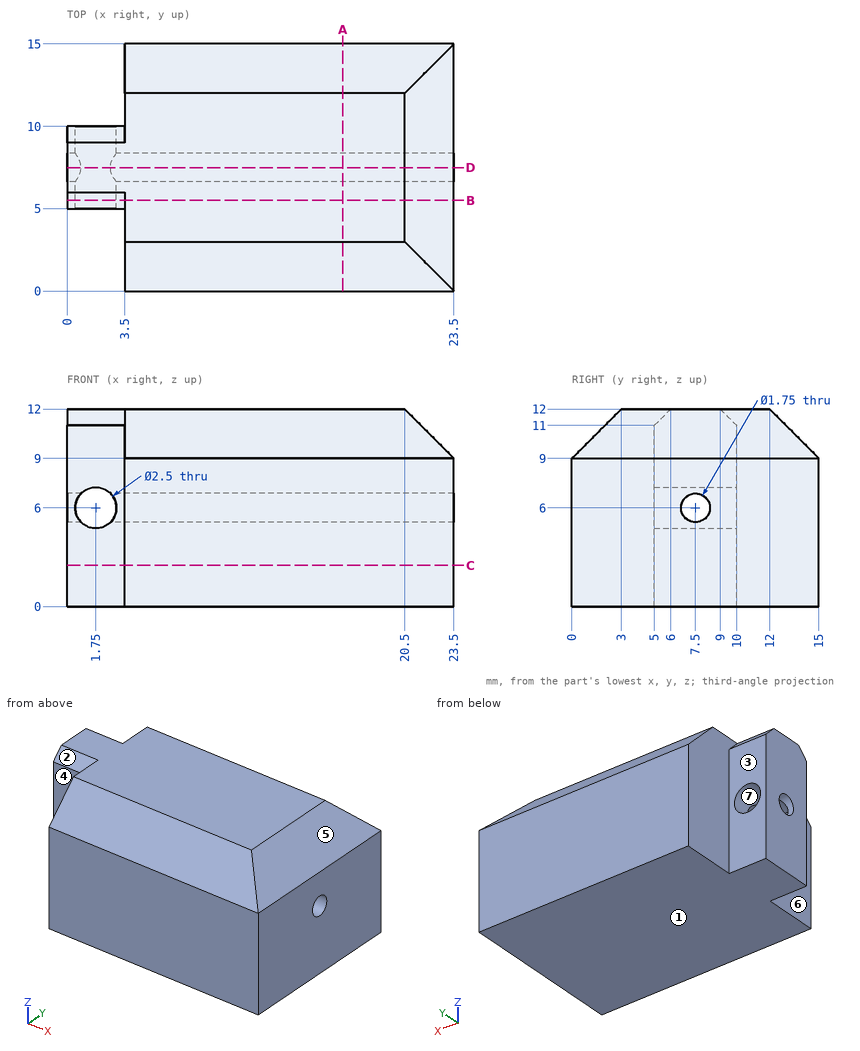
For this review, use the dimensioned drawing (mm, ordinates from the lowest corner) and the shaded views. A direction names the side the tool comes from. Coordinates: 2 decimals unless noted, no trailing zeros. Order: outer loops, then holes, each group sorted by start corner. A loop starts at its lowest first (then second) coordinate and runs counter-clockwise, first axis right, second up. Notation, with made-up numbers: (-0.75, 15) - (28.25, 15) arc R12 ccw to (28.25, 23) - close; hole circle Ø4 at (8.25, 65.5). An arc over 180 degrees is marked (long way). Answer as a JSON object with one key per item and string values. Group by question number.
1. For the marked faces 1, 2 and 3, list the 3-axis set-ups (+Z, -Z, +X, -X, +Y, -Y) from which the entire face can be reached by the end or side of a thin tool; tool diameter is ignored.
2. For probe 1 along Y at (x, z) = (15, 6) (3 decimals); probe 2 along Z at (x, y) = (0.2, 7.5) (3 decimals); probe 3 along X at (y, z) = (8.65, 6), list the stretches that pass through material, from the lowest coordinate up.
3. We need section A-A on x = 16.75. State the section outline as (y, z) points (3 decimals), then the cut area to 3 significant figures.
4. We need section C-C on z = 2.5. State the section outline as (x, y) points.
5. We need section B-B on y = 5.5. State the section outline as (x, z) points, then the cut area to 3 significant figures.
6. Clearance check with flat-ended pins moving along their axes: P1, Ø1.8, axis at y = 4, z = 7, coming from the -X side; P2, Ø1.4, axis at y = 7.5, z = 6, coming from the -X side; P3, Ø1.8, axis at x = 1.5, z = 5, coming from the -Y side. State where each tip first meets the part, or that it passes through.
7. The part is to be moulded in two halves that separate along X. For the marked faces 4, 5, 6 and 7, say which applies: pulls with the +X half, pulls with the -X half, needs draft (parallel to the pull), parting line crosses it, or undercut.
8. We need section D-D on y = 7.5. State the section outline as (x, z) points (3 decimals).
Final values:
{
 "1": {"face 1": "-Z, +X, -X, +Y, -Y", "face 2": "+Z, -X, -Y", "face 3": "+Z, -Z, -X, +Y"},
 "2": {"probe 1": "0 to 6.625, 8.375 to 15", "probe 2": "0 to 5.125, 6.875 to 12", "probe 3": "0 to 0.5, 3 to 23.5"},
 "3": {"outline": "(0, 0) - (15, 0) - (15, 9) - (12, 12) - (3, 12) - (0, 9) - close; hole circle Ø1.75 at (7.5, 6)", "area": "169 mm²"},
 "4": {"outline": "(0, 5) - (3.5, 5) - (3.5, 0) - (23.5, 0) - (23.5, 15) - (3.5, 15) - (3.5, 10) - (0, 10) - close"},
 "5": {"outline": "(0, 0) - (23.5, 0) - (23.5, 9) - (20.5, 12) - (3.5, 12) - (3.5, 11.5) - (0, 11.5) - close; hole circle Ø2.5 at (1.75, 6)", "area": "271 mm²"},
 "6": {"P1": "x = 3.5", "P2": "through", "P3": "y = 5"},
 "7": {"face 4": "needs draft", "face 5": "pulls with the +X half", "face 6": "pulls with the -X half", "face 7": "undercut"},
 "8": {"outline": "(0, 0) - (23.5, 0) - (23.5, 5.125) - (2.643, 5.125) arc R1.25 cw to (0.857, 5.125) - (0, 5.125) - close; (0, 6.875) - (0.857, 6.875) arc R1.25 cw to (2.643, 6.875) - (23.5, 6.875) - (23.5, 9) - (20.5, 12) - (0, 12) - close"}
}
